Input: part model. Units: mm. Frame: model coordinates. A direction names the side the tool comes from. Give positions to 0.01 mm unless a question says otherwise; leave off trailing zeros. Loops run counter-clockwise (first coordinate to the right, second up) from the corner with the lowest first, then second, coordinate; pieces in that order, holes last. Notation, with made-up numbers: M 81.25,41 L 122.25,41 A7 ccw 122.25,53 Z; hole C 10,36 d4. An arc over 180 degrees is marked long. Use CSV: the item, a comma, the result in double quotes. Start each with the question number.
Q1. Material intervals for line 1 along Y through (x, z) = (-6.75, 4.75); line 2 along X through (y, z) = (-6.65, 4); line 3 along Y through (x, z) = (-1.5, 7.75), sorted ascending.
Q2. Section C-C, the plane z = 7. Output: boundary loops of the cut face in (x, y), plus the area to 3 significant figures.
Q3. Pull-direction query (Z, two-part tool) for faces 4 (the cylindrical face through (-4.9, -0.9, 2.5)), 5 (the cylindrical face through (-3.62, -7.11, 3.31)), 6 (the flat face through (-5, -7, 0)), 7 (the flat face through (-6.45, -1, 6)); classes: released by +Z, released by -Z, zero draft, split by the parting line, or undercut.
Q4. Section A-A, the plane x = -3.75. Output: boundary loops of the cut face in (y, z), plus the area to 3 significant figures.
Q5. Pin query (flat end, axial travel): pin 1 (2.5 mm diameter, centred on x = -1.75, y = -6.25, fed in from -Z); pin 2 (1.2 mm diameter, centred on x = -8.15, y = -6.25, fed in from -Z). Return the tip coordinate at first contact, or that it passes through.
Q6. Section D-D, the plane x = -5.25. Output: boundary loops of the cut face in (y, z).
Q7. Section B-B, the plane y = -2. Output: boundary loops of the cut face in (x, z).
Q8. Reachability of faces 1 (the flat face through (-1.75, -4, 4)), 2 (the flat face through (-5, 0, 2)), 3 (the flat face through (-3.45, -1, 6)) from +Z, -Z, +X, -X, +Y, -Y: full face, straight path, thin tool, end or side. Return the list, or none.
Autodesk Fusion 360 part; units mm, degrees
sketch "Sketch1" plane through (0, 0, 0) normal (0, 0, 1) x (1, 0, 0) in component "Prusa Expansion Joint"
  line L0 (-9.15, -8) -> (-0.75, -8)
  line L1 (0, -7.25) -> (0, -0.75)
  line L2 (-0.75, 0) -> (-9.15, 0)
  line L3 (-9.9, -0.75) -> (-9.9, -7.25)
  line L4 (-8.15, -6.25) -> (-1.75, -6.25)
  line L5 (-1.75, -6.25) -> (-1.75, -1.75)
  line L6 (-1.75, -1.75) -> (-8.15, -1.75)
  line L7 (-8.15, -1.75) -> (-8.15, -6.25)
  circle A0 centre (-1.75, -1.75) radius 0.75
  circle A1 centre (-8.15, -6.25) radius 0.75
  circle A2 centre (-8.15, -1.75) radius 0.75
  circle A3 centre (-1.75, -6.25) radius 0.75
  line L8 (-9.15, 0) -> (-9.9, -0.75)
  line L9 (-9.9, -7.25) -> (-9.15, -8)
  line L10 (0, -7.25) -> (-0.75, -8)
  line L11 (0, -0.75) -> (-0.75, 0)
  line L12 (0, -0.75) -> (0, 0) construction
  line L13 (0, 0) -> (-0.75, 0) construction
  dimension "d4" = 1.5
  dimension "d5" = 1.5
  dimension "d6" = 1.5
  dimension "d7" = 1.5
  dimension "d15" = 1.75
  dimension "d16" = 1.75
  dimension "d17" = 1.75
  dimension "d18" = 1.75
  dimension "d26" = 135
  dimension "d27" = 135
  dimension "d30" = 8
  dimension "d31" = 9.9
  dimension "d32" = 0.75
extrude "Extrude1" add sketch "Sketch1" along normal blind 8 in component "Prusa Expansion Joint"
hole "Hole1" at (-4.95, -8, 4) direction (0, 1, 0) diameter 3 depth 8 tip angle 180 in component "Prusa Expansion Joint"
sketch "Sketch2" plane through (0, 0, 0) normal (0, 1, 0) x (1, 0, 0) in component "Prusa Expansion Joint"
  line L0 (-3.45, -4) -> (-6.45, -4)
  line L1 (-6.45, -4) -> (-6.45, -8)
  line L2 (-6.45, -8) -> (-3.45, -8)
  line L3 (-3.45, -8) -> (-3.45, -4)
  dimension "d33" = 3
  dimension "d34" = 4
  dimension "d35" = 4
  dimension "d36" = 3.45
extrude "Extrude2" cut sketch "Sketch2" against normal blind 1.75 in component "Prusa Expansion Joint"
component "Prusa Expansion Joint" placed x (1, 0, 0) y (0, 1, 0) z (0, 0, 1) at (0, 0, 0)
equation "d4 = ( 0.75 * 2 ) * 1 mm"
equation "d25 = ( 9.9 / 2 ) * 1 mm"
equation "d26 = 45 deg + 45 deg + 45 deg"
equation "d36 = ( ( 9.9 / 2 ) * 1 mm ) - 1.5 mm"
A:
1,line 1,"-8 to -6.25, -1.75 to 0"
1,line 2,"-9.9 to -8.78, -7.52 to -6.45, -3.45 to -2.38, -1.12 to 0"
1,line 3,"-8 to -6.96, -5.54 to -2.46, -1.04 to 0"
2,outline,"M -9.9,-7.25 L -9.15,-8 L -0.75,-8 L 0,-7.25 L 0,-0.75 L -0.75,0 L -3.45,0 L -3.45,-1.75 L -2.5,-1.75 A0.75 cw long -1.75,-2.5 L -1.75,-5.5 A0.75 cw long -2.5,-6.25 L -7.4,-6.25 A0.75 cw long -8.15,-5.5 L -8.15,-2.5 A0.75 cw long -7.4,-1.75 L -6.45,-1.75 L -6.45,0 L -9.15,0 L -9.9,-0.75 Z"
2,area,"38.7 mm^2"
3,face 4,"released by +Z"
3,face 5,"undercut"
3,face 6,"released by -Z"
3,face 7,"zero draft"
4,outline,"M -8,0 L -6.25,0 L -6.25,3.1 L -8,3.1 Z; M -8,4.9 L -6.25,4.9 L -6.25,8 L -8,8 Z; M -1.75,0 L 0,0 L 0,3.1 L -1.75,3.1 Z"
4,area,"16.3 mm^2"
5,pin 1,"z = 0"
5,pin 2,"through"
6,outline,"M -8,0 L -6.25,0 L -6.25,2.53 L -8,2.53 Z; M -8,5.47 L -6.25,5.47 L -6.25,8 L -8,8 Z; M -1.75,0 L 0,0 L 0,2.53 L -1.75,2.53 Z"
7,outline,"M -9.9,0 L -8.86,0 L -8.86,8 L -9.9,8 Z; M -1.04,0 L 0,0 L 0,8 L -1.04,8 Z"
8,face 1,"+Z, -Z"
8,face 2,"+Z, -Z, +X, -X, +Y"
8,face 3,"+Z, +Y"
